Source: CAD feature listing. Evaluate the final solid. Frame: model axes, mm. A direction names the side the tool comes from. Round coordinates to 2 decimals unless told otherwise and drop trailing zeros. Order: outer loops, then holes, each group sorted by start corner. A loop starts at its lowest first (then second) coordinate and runs counter-clockwise, first axis right, second up. Notation, with made-up numbers: (56.25, 43.5) -> (87.25, 43.5) arc R12 cw to (87.25, 57.5) -> close; hole circle Ø8 at (30.5, 78). An arc over 180 degrees is marked (long way). Write item = value, one per line. Start each with the question number.
(1) Cut plane B-B on z = -12.5. Return the cut outline in (x, y), then the cut area to 3 significant figures.
(2) Draft query along X for faces 6 (the face through (0, 2, -10)), 7 (the face through (10, 2, 0)), 8 (the face through (12.77, 10.14, -8.85)). Return one class per face: released by +X, released by -X, zero draft, split by the parting line, or undercut.
(3) Ray query, line 1 (X direction, y = 13, z = -10); line 2 (Z direction, x = 10, y = 11.5); line 3 (Y direction, x = 18, z = -1.5). Return the intervals inside material, ascending.
(4) Cut plane D-D on x = 11.5. Return the cut outline in (y, z).
(5) Cut plane C-C on y = 2. Return the cut outline in (x, z), then the cut area to 3 significant figures.
(6) Cut plane A-A on x = 4. Return the cut outline in (y, z).
(7) Reachability of faces 1 (the face through (2, 5, -18)), 2 (the face through (18, 5, -2)), 3 (the face through (2, 13, -4)), 4 (the face through (2, 5, -2)), 5 (the face through (18, 5, -18)) from +Z, -Z, +X, -X, +Y, -Y: full face, straight path, thin tool, end or side. Return the list, or none.
(8) Contact query for flat-ended pins moving along their axis: pin 1 Ø3 at (x, y) = (8.5, 10) entering from -Z; pin 2 Ø2 at (x, y) = (17.5, 15) entering from -Z; pin 3 Ø6 at (y, z) = (11.5, -13.5) entering from +X; pin 4 Ø1 at (y, z) = (11.5, -16.5) entering from -X. Output: stop coordinate, or through.
from build123d import *

# Parameters (mm, degrees)
SKETCH1_W           = 20
SKETCH1_H           = 20
BOSS_EXTRUDE1_DEPTH = 20
SKETCH2_OUTSIDE_W   = 28.928
SKETCH2_OUTSIDE_H   = 28.928
SKETCH2_OUTSIDE_R   = 10
CUT_EXTRUDE1_DEPTH  = 15
SKETCH3_R           = 3
CUT_EXTRUDE2_DEPTH  = 21


with BuildPart() as part:
    # Sketch1 → Boss-Extrude1 (new body)
    with BuildSketch(Plane(origin=(0, 0, 0), x_dir=(1, 0, 0), z_dir=(0, 1, 0))):
        with Locations((10, 10)):
            Rectangle(SKETCH1_W, SKETCH1_H)
    extrude(amount=BOSS_EXTRUDE1_DEPTH)

    # Sketch2 outside → Cut-Extrude1 (cut)
    with BuildSketch(Plane(origin=(0, 20, 0), x_dir=(1, 0, 0), z_dir=(0, 1, 0))):
        with Locations((10, 10)):
            Rectangle(SKETCH2_OUTSIDE_W, SKETCH2_OUTSIDE_H)
        with Locations((10, 10)):
            Circle(SKETCH2_OUTSIDE_R, mode=Mode.SUBTRACT)
    extrude(amount=-CUT_EXTRUDE1_DEPTH, mode=Mode.SUBTRACT)

    # Sketch3 → Cut-Extrude2 (cut, through all)
    with BuildSketch(Plane(origin=(0, 20, 0), x_dir=(1, 0, 0), z_dir=(0, 1, 0))):
        with Locations((10, 10)):
            Circle(SKETCH3_R)
    extrude(amount=-CUT_EXTRUDE2_DEPTH, mode=Mode.SUBTRACT)


solid = part.part
Evaluation:
q1.outline = (0, 0) -> (8.34, 0) -> (8.34, 20) -> (0.32, 20) -> (0.32, 5) -> (0, 5) -> close; (11.66, 0) -> (20, 0) -> (20, 5) -> (19.68, 5) -> (19.68, 20) -> (11.66, 20) -> close
q1.area = 324 mm^2
q2.face_6 = released by -X
q2.face_7 = zero draft
q2.face_8 = undercut
q3.line_1 = 0 to 7, 13 to 20
q3.line_2 = -20 to -13, -7 to 0
q3.line_3 = 0 to 5
q4.outline = (0, -20) -> (5, -20) -> (5, -19.89) -> (20, -19.89) -> (20, -12.6) -> (0, -12.6) -> close; (0, -7.4) -> (20, -7.4) -> (20, -0.11) -> (5, -0.11) -> (5, 0) -> (0, 0) -> close
q5.outline = (0, -20) -> (20, -20) -> (20, 0) -> (0, 0) -> close; hole circle Ø6 at (10, -10)
q5.area = 372 mm^2
q6.outline = (0, -20) -> (5, -20) -> (5, -18) -> (20, -18) -> (20, -2) -> (5, -2) -> (5, 0) -> (0, 0) -> close
q7.face_1 = -Z, -X, +Y
q7.face_2 = +Z, +X, +Y
q7.face_3 = +Y
q7.face_4 = +Z, -X, +Y
q7.face_5 = -Z, +X, +Y
q8.pin_1 = -20
q8.pin_2 = -17.6
q8.pin_3 = 19.99
q8.pin_4 = 2
